```python
from build123d import *

# Parameters (mm, degrees)
SKETCH1_R           = 9.149999998
BOSS_EXTRUDE1_DEPTH = 64.5
SKETCH2_R           = 7.15
CUT_EXTRUDE1_DEPTH  = 0.2
FILLET1_R           = 0.5


with BuildPart() as part:
    # Sketch1 → Boss-Extrude1 (new body)
    with BuildSketch(Plane.XY):
        Circle(SKETCH1_R)
    extrude(amount=BOSS_EXTRUDE1_DEPTH)

    # Sketch2 → Cut-Extrude1 (cut)
    with BuildSketch(Plane.XY):
        Circle(SKETCH2_R)
    extrude(amount=CUT_EXTRUDE1_DEPTH, mode=Mode.SUBTRACT)

    # Sketch3 → Cut-Revolve1 (revolve, cut)
    with BuildSketch(Plane(origin=(0, 0, 0), x_dir=(1, 0, 0), z_dir=(0, 1, 0))):
        Polygon((-8.149999999, -64.2), (-8.149999999, -63.700000001), (-4.799999999, -63.700000001), (-3.999999999, -64.5), (-6.650000001, -64.5), (-6.650000001, -64.35), (-5.649999999, -64.35), (-5.649999999, -64.2), align=None)
    revolve(axis=Axis((0, 0, 64.835920194), (0, 0, -1)), mode=Mode.SUBTRACT)

    # Fillet1
    fillet1_edges = [part.edges().sort_by_distance(p)[0] for p in [
        (-9.149999998, 0, 0),
        (-9.149999998, 0, 64.5),
    ]]
    fillet(fillet1_edges, radius=FILLET1_R)


solid = part.part
```
For this review, take the finished solid that the model builds, in its own axes (mm). A direction names the side the tool comes from. Round coordinates to 2 decimals unless told otherwise and drop trailing zeros. Order: outer loops, then holes, each group sorted by start corner. A loop starts at its lowest first (then second) coordinate and runs counter-clockwise, first axis right, second up.
Q1. We need section A-A, the plane z = 60. Give the boundary of the cut face in (x, y), plus the area to 3 significant figures.
Findings below:
outline: circle Ø18.3 at (0, 0)
area: 263 mm2
Q2. Mouldability with a two-part tool opening along Z and no side actions: class faces 4 (the cylindrical face through (-7.774, 2.448, 63.947)), 5 (the flat face through (-5.2, 5.2, 0)), 6 (the flat face through (2.5, -6.4, 64.5)) as pulls with the +Z half, pulls with the -Z half, needs draft (parallel to the pull), parting line crosses it, or undercut.
Findings below:
face 4: undercut
face 5: pulls with the -Z half
face 6: pulls with the +Z half
Q3. Insertion check: P1, Ø8, axis at x = 0, y = -0.5, coming from the -Z side; P2, Ø4, axis at x = -6, z = 48, coming from the -Y side; P3, Ø10, axis at x = -6, z = 45.5, coming from the +Y side. Each pin has a flat end and moves straight along its axis. Give the tip position at first contact, or say it passes through.
Findings below:
P1: stops at z = 0.2
P2: stops at y = -8.23
P3: stops at y = 9.1
Q4. Machinability: for faces 1 (the flat face through (0, 0, 64.5)), 2 (the flat face through (-4, -4, 63.7)), 3 (the flat face through (0, 0, 0.2)), which of the approach directions +Z, -Z, +X, -X, +Y, -Y give a long, thin tool a straight path to every point of the face, cutting with its end or side? Answer none if there is none.
Findings below:
face 1: +Z, +X, -X, +Y, -Y
face 2: none
face 3: -Z
Q5. Wall thickness on line 1 (Z direction, x = -1.75, y = -7.25); line 2 (Y direction, x = 0.5, z = 61.5); line 3 (Y direction, x = 0, z = 64.3): over which ranges is each line inside the solid? List them lowest first.
Findings below:
line 1: z = 0 to 63.7, 64.2 to 64.5
line 2: y = -9.14 to 9.14
line 3: y = -9.05 to -5.65, -4.2 to 4.2, 5.65 to 9.05
